Geometry: see drawing. Coordinates: mm, zero at the bounding-box minimum. Give positions to 0.01 mm unless a question says otherwise; leave off trailing zeros. Write each loop counter-clockwise with the first axis right and the second up, starting at its lowest first coordinate (ties: lowest second). Pieces come first, ordered by that corner, then holes. Notation, with made-up numbers: (44.5, 12.5) -> (89.5, 12.5) arc R27 cw to (89.5, 42.5) -> close; hole circle Ø2 at (38.5, 57.25). An arc over 180 degrees is marked (long way). Answer as a JSON object with one key per item and string values. Group by question number.
Item 1: Section query D-D on x = 4.28. Return the cut outline in (y, z), plus the area to 3 significant figures.
Item 2: Section query B-B on y = 18.5. Return the cut outline in (x, z).
Item 3: First-contact query: pin 1 Ø5.5 at (x, z) = (12, 7.5) entering from -Y. Flat tip, straight axial feed; report the tip coordinate or a pass-through.
Item 4: Section query C-C on z = 1.75. Return the cut outline in (x, y).
Item 5: Section query A-A on x = 11.9. Return the cut outline in (y, z), plus the area to 3 significant figures.
Item 6: Ray query, probe 1 along Y at (x, z) = (11.9, 7); probe 2 along Y at (x, z) = (10.5, 6.75); probe 3 along X at (y, z) = (20.5, 2.25). Return the intervals inside material, ascending. Write a range as from..to.
Item 7: Pull-direction query (Y, two-part tool) for the marked faces 1, 2 and 3; classes: pulls with the +Y half, pulls with the -Y half, needs draft (parallel to the pull), parting line crosses it, or undercut.
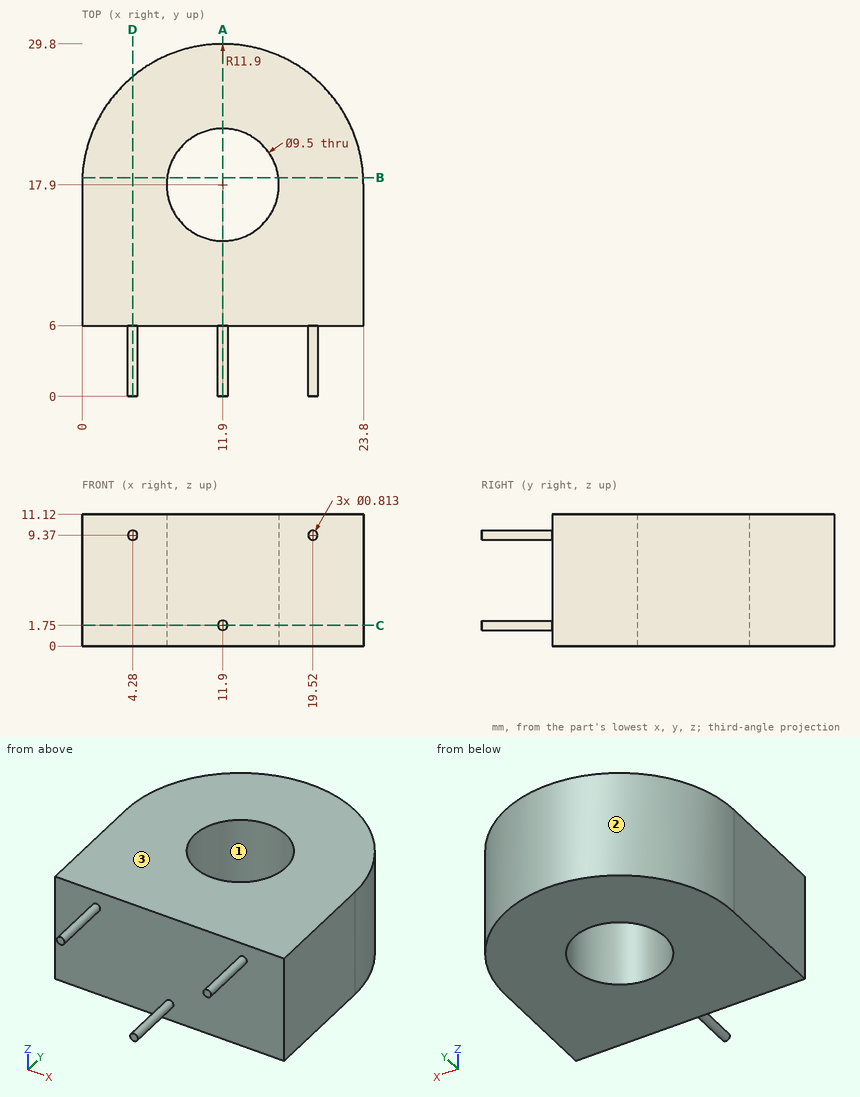
Worked answers:
{
 "1": {"outline": "(0, 8.96) -> (6, 8.96) -> (6, 0) -> (27.04, 0) -> (27.04, 11.12) -> (6, 11.12) -> (6, 9.78) -> (0, 9.78) -> close", "area": "239 mm^2"},
 "2": {"outline": "(0.02, 0) -> (7.19, 0) -> (7.19, 11.12) -> (0.02, 11.12) -> close; (16.61, 0) -> (23.78, 0) -> (23.78, 11.12) -> (16.61, 11.12) -> close"},
 "3": {"pin 1": "y = 6"},
 "4": {"outline": "(0, 6) -> (11.49, 6) -> (11.49, 0) -> (12.31, 0) -> (12.31, 6) -> (23.8, 6) -> (23.8, 17.9) arc R11.9 ccw to (0, 17.9) -> close; hole circle Ø9.5 at (11.9, 17.9)"},
 "5": {"outline": "(0, 1.34) -> (6, 1.34) -> (6, 0) -> (13.15, 0) -> (13.15, 11.12) -> (6, 11.12) -> (6, 2.16) -> (0, 2.16) -> close; (22.65, 0) -> (29.8, 0) -> (29.8, 11.12) -> (22.65, 11.12) -> close", "area": "164 mm^2"},
 "6": {"probe 1": "6..13.15, 22.65..29.8", "probe 2": "6..13.36, 22.44..29.72", "probe 3": "0.29..7.92, 15.88..23.51"},
 "7": {"face 1": "undercut", "face 2": "pulls with the +Y half", "face 3": "needs draft"}
}
